Source: CAD feature listing. Evaluate the final solid. Frame: model axes, mm. A direction names the side the tool comes from. Coordinates: 2 decimals unless noted, no trailing zeros. Order: outer loops, then holes, each group sorted by start corner. A loop starts at its lowest first (then second) coordinate and runs counter-clockwise, first axis right, second up.
```python
from build123d import *

# Parameters (mm, degrees)
SKETCH_2_R          = 1.5
CUT_EXTRUDE_1_DEPTH = 20.923855049
EXTRUDE_START       = 1
EXTRUDE_1_DEPTH     = 1


with BuildPart() as part:
    # ｽｹｯﾁ1 → 回転1 (revolve)
    with BuildSketch(Plane.XY):
        with BuildLine():
            Line((0, 0), (13.6, 0))
            Line((13.6, 0), (13.6, 1))
            Line((13.6, 1), (11.6, 1))
            ThreePointArc((11.6, 1), (10, 2.6), (11.6, 4.2))
            Line((11.6, 4.2), (13.6, 4.2))
            Line((13.6, 4.2), (13.6, 5.2))
            Line((13.6, 5.2), (0, 5.2))
            Line((0, 5.2), (0, 0))
        make_face()
    revolve(axis=Axis((0, 0, 0), (0, 1, 0)))

    # ｽｹｯﾁ2 → ｶｯﾄ - 押し出し1 (cut, through all)
    with BuildSketch(Plane(origin=(0, 5.2, 0), x_dir=(1, 0, 0), z_dir=(0, 1, 0))):
        with Locations(Location((0, 0, 0), (0, 0, 180))):
            Circle(SKETCH_2_R)
    extrude(amount=-CUT_EXTRUDE_1_DEPTH, mode=Mode.SUBTRACT)

    # ｽｹｯﾁ3 → ﾎﾞｽ - 押し出し1 (add)
    with BuildSketch(Plane(origin=(0, 5.2, 0), x_dir=(1, 0, 0), z_dir=(0, 1, 0)).offset(EXTRUDE_START)):
        with BuildLine():
            Line((3, 13.264991519), (3, -13.264991519))
            ThreePointArc((3, -13.264991519), (4.011896667, -12.99479454), (5, -12.647529403))
            Line((5, -12.647529403), (5, 12.647529403))
            ThreePointArc((5, 12.647529403), (4.011896667, 12.99479454), (3, 13.264991519))
        make_face()
        with BuildLine():
            Line((-5, 12.647529403), (-5, -12.647529403))
            ThreePointArc((-5, -12.647529403), (-4.011896667, -12.99479454), (-3, -13.264991519))
            Line((-3, -13.264991519), (-3, 13.264991519))
            ThreePointArc((-3, 13.264991519), (-4.011896667, 12.99479454), (-5, 12.647529403))
        make_face()
    extrude(amount=-EXTRUDE_1_DEPTH)


solid = part.part
```
1. Section query A-A, the plane z = 0. Output: boundary loops of the cut face in (x, y).
2. Section query C-C, the plane y = 3.75. Output: boundary loops of the cut face in (x, z), plus the area to 3 significant figures.
3. Material intervals for line 1 along Y through (x, z) = (-10.5, 6.5); line 2 along X through (y, z) = (5.75, 8.25); line 3 along Z through (x, y) = (0, 4.25), sorted ascending.
4. Section query B-B, the plane x = 0. Output: boundary loops of the cut face in (y, z).
5. Contact query for flat-ended pins moving along their axis: P1, Ø9.5, axis at x = 8.5, z = 0, coming from the +Y side; P2, Ø0.5, axis at y = 5.5, z = 6, coming from the +X side; P3, Ø3, axis at x = 7, y = 4.5, coming from the +Z side; P4, Ø1.5, axis at x = 7.5, y = 2, coming from the -Z side. Output: stop coordinate, or through.
6. Access query for faces 1 (the flat face through (-11.02, 4.2, -4.09)), 2 (the cylindrical face through (-2.948, 0.507, 13.277)), 3 (the flat face through (8, 5.2, 0)), 4 (the flat face through (-2, 5.2, 0)), 5 (the flat face through (-5, 6, 0)). Directions: +Z, -Z, +X, -X, +Y, -Y. A direction counts if a zero-diameter tool reaches every point of the face in a straight line with its end or side. Return the directions, or none.
7. Draft query along Y for faces 6 (the flat face through (11.02, 1, -4.09)), 7 (the flat face through (0, 0, 3)), 8 (the flat face through (4, 6.2, 0)), 9 (the flat face through (-3, 6, 0)). Return one class per face: +Y half, -Y half, draft (parallel to the pull), parting line (faces both ways), or undercut.
8. Section query D-D, the plane x = 12.25. Output: boundary loops of the cut face in (y, z).
Answer key:
1. outline: (-13.6, 0) - (-1.5, 0) - (-1.5, 5.2) - (-3, 5.2) - (-3, 6.2) - (-5, 6.2) - (-5, 5.2) - (-13.6, 5.2) - (-13.6, 4.2) - (-11.6, 4.2) arc R1.6 cw to (-11.6, 1) - (-13.6, 1) - close; (1.5, 0) - (13.6, 0) - (13.6, 1) - (11.6, 1) arc R1.6 cw to (11.6, 4.2) - (13.6, 4.2) - (13.6, 5.2) - (5, 5.2) - (5, 6.2) - (3, 6.2) - (3, 5.2) - (1.5, 5.2) - close
2. outline: circle Ø20.98 at (0, 0); hole circle Ø3 at (0, 0)
2. area: 338 mm2
3. line 1: y = 0 to 1, 4.2 to 5.2
3. line 2: x = -5 to -3, 3 to 5
3. line 3: z = -13.6 to -1.5, 1.5 to 13.6
4. outline: (0, -13.6) - (1, -13.6) - (1, -11.6) arc R1.6 cw to (4.2, -11.6) - (4.2, -13.6) - (5.2, -13.6) - (5.2, -1.5) - (0, -1.5) - close; (0, 1.5) - (5.2, 1.5) - (5.2, 13.6) - (4.2, 13.6) - (4.2, 11.6) arc R1.6 cw to (1, 11.6) - (1, 13.6) - (0, 13.6) - close
5. P1: stops at y = 6.2
5. P2: stops at x = 5
5. P3: stops at z = 12.44
5. P4: stops at z = -7.85
6. face 1: none
6. face 2: +Y, -Y
6. face 3: +Z, -Z, +X, +Y
6. face 4: +Z, -Z, +Y
6. face 5: +Z, -Z, -X, +Y
7. face 6: undercut
7. face 7: -Y half
7. face 8: +Y half
7. face 9: draft
8. outline: (0, -5.91) - (1, -5.91) - (1, 5.91) - (0, 5.91) - close; (4.2, -5.91) - (5.2, -5.91) - (5.2, 5.91) - (4.2, 5.91) - close
